Geometry: final body of the model. Coordinates: model frame, mm. Give positions to 0.01 mm unless a question says otherwise; leave off trailing zeros. Loops run counter-clockwise (first coordinate to the right, second up) from the corner with the lowest first, then second, coordinate; pieces in that order, holes last.
1. Material intervals for line 1 along X through (y, z) = (-1.5, 22); line 2 along X through (y, z) = (-0.75, 18); line 3 along Y through (x, z) = (-9.5, -17), sorted ascending.
2. Section A-A, the plane z = 51.5. Output: boundary loops of the cut face in (x, y).
3. Section C-C, the plane y = -4.75. Output: boundary loops of the cut face in (x, z).
4. First-contact query: P1, Ø1.5, axis at x = -1.5, z = -53, coming from the -Y side; P2, Ø4, axis at x = -15, z = 13, coming from the -Y side; P3, Ø5.5, axis at x = -3.5, z = 57.5, coming from the -Y side. Flat tips, straight axial feed; report the tip coordinate or a pass-through.
5. Section D-D, the plane x = -11. Output: boundary loops of the cut face in (y, z), then the cut area to 3 significant figures.
6. Section B-B, the plane x = -3.75. State how many separate pieces and enclosed holes the cut face has, then the cut area to 3 significant figures.
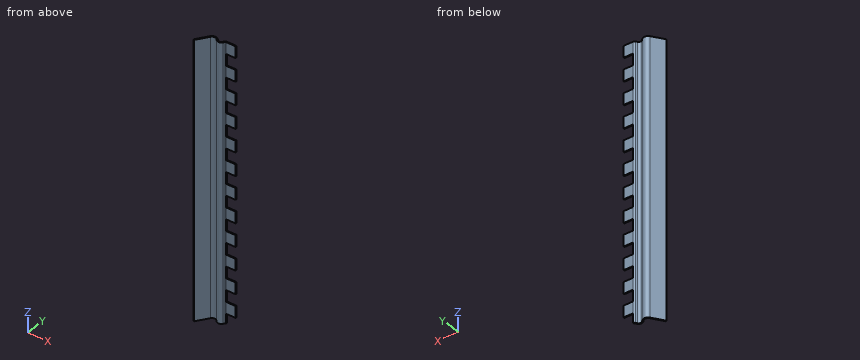
from build123d import *

# Parameters (mm, degrees)
BOSS_EXTRUDE1_DEPTH = 71.5
SKETCH3_W           = 5
SKETCH3_H           = 6
CUT_EXTRUDE1_DEPTH  = 74.85295489
LPATTERN1_COUNT     = 12
LPATTERN1_PITCH     = 12


with BuildPart() as part:
    # Sketch1 → Boss-Extrude1 (new, symmetric)
    with BuildSketch(Plane.XY):
        with BuildLine():
            Line((0, 0), (-5, 0))
            ThreePointArc((-5, 0), (-5.468268863, -0.11641397), (-5.827511651, -0.438551456))
            Line((-5.827511651, -0.438551456), (-6.324130952, -1.170512135))
            ThreePointArc((-6.324130952, -1.170512135), (-7.565398428, -1.828339319), (-8.806665905, -1.170512135))
            Line((-8.806665905, -1.170512135), (-8.856963859, -1.096378639))
            ThreePointArc((-8.856963859, -1.096378639), (-10.925742986, 0), (-12.994522113, -1.096378639))
            Line((-12.994522113, -1.096378639), (-17, -7))
            Line((-17, -7), (-16.586244175, -7.280724272))
            Line((-16.586244175, -7.280724272), (-12.580766288, -1.377102912))
            ThreePointArc((-12.580766288, -1.377102912), (-10.925742986, -0.5), (-9.270719684, -1.377102912))
            Line((-9.270719684, -1.377102912), (-9.22042173, -1.451236407))
            ThreePointArc((-9.22042173, -1.451236407), (-7.565398428, -2.328339319), (-5.910375127, -1.451236407))
            Line((-5.910375127, -1.451236407), (-5.413755825, -0.719275728))
            ThreePointArc((-5.413755825, -0.719275728), (-5.234134431, -0.558206985), (-5, -0.5))
            Line((-5, -0.5), (0, -0.5))
            Line((0, -0.5), (0, 0))
        make_face()
    extrude(amount=BOSS_EXTRUDE1_DEPTH, both=True)

    # Sketch3 → Cut-Extrude1 (cut, through all)
    with BuildSketch(Plane(origin=(0, 0, 0), x_dir=(1, 0, 0), z_dir=(0, 1, 0))):
        with Locations((-2.5, -62.5)):
            Rectangle(SKETCH3_W, SKETCH3_H)
    cut_extrude1 = extrude(amount=-CUT_EXTRUDE1_DEPTH, mode=Mode.SUBTRACT)

    # LPattern1: Cut-Extrude1 ×12
    with Locations(*[(0, 0, -i * LPATTERN1_PITCH) for i in range(1, LPATTERN1_COUNT)]):
        add(cut_extrude1, mode=Mode.SUBTRACT)


solid = part.part
Answers below:
1. line 1: x = -13.27 to -12.66, -9.19 to -8.5, -6.63 to -5.94
1. line 2: x = -12.71 to -11.89, -9.96 to -9.14, -6.04 to -5.43
1. line 3: y = -1.1 to -0.45
2. outline: (-17, -7) - (-16.59, -7.28) - (-12.58, -1.38) arc R2 cw to (-9.27, -1.38) - (-9.22, -1.45) arc R2 ccw to (-5.91, -1.45) - (-5.41, -0.72) arc R0.5 cw to (-5, -0.5) - (-5, 0) arc R1 ccw to (-5.83, -0.44) - (-6.32, -1.17) arc R1.5 cw to (-8.81, -1.17) - (-8.86, -1.1) arc R2.5 ccw to (-12.99, -1.1) - close
3. outline: (-15.47, -71.5) - (-14.87, -71.5) - (-14.87, 71.5) - (-15.47, 71.5) - close
4. P1: stops at y = -0.5
4. P2: stops at y = -7.28
4. P3: stops at y = -1.83
5. outline: (-0.5, -71.5) - (0, -71.5) - (0, 71.5) - (-0.5, 71.5) - close
5. area: 71.5 mm2
6. separate pieces: 12
6. enclosed holes: 0
6. area: 36.0 mm2
